Check sheet for the modelled part. Datum: model origin and axes. Units: mm. Face numbers are marked on the shaded views. A direction names the side the tool comes from. Coordinates: 2 decimals unless noted, no trailing zeros. Order: outer loops, then holes, each group sorted by start corner. A loop starts at its lowest first (then second) coordinate and runs counter-clockwise, first axis right, second up.
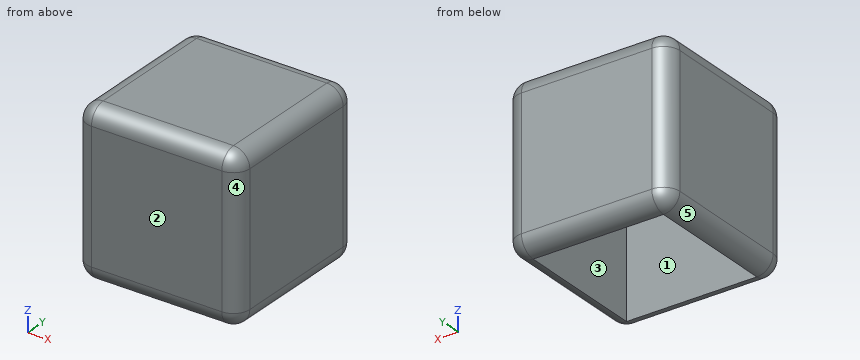
from build123d import *

# Parameters (mm, degrees)
F0_W      = 101.6
F0_H      = 101.6
F1_DEPTH  = 101.6
F2_R      = 50.8
F3_DEPTH  = 101.6
F9_W      = 101.6
F9_H      = 101.6
F10_DEPTH = 101.6
F11_R     = 10.16
F12_W     = 81.28
F12_H     = 81.28
F14_DEPTH = 88.9


# Not quite as in the source:
# - a feature of the source that left no trace in its solid (it failed there, or was rolled back) is left out


with BuildPart() as f1:
    # F0 (on Top) → F1 (new body)
    with BuildSketch(Plane.XY):
        Rectangle(F0_W, F0_H)
    extrude(amount=F1_DEPTH)


with BuildPart() as f3:
    # F2 (on Top) → F3 (new body)
    with BuildSketch(Plane.XY):
        Circle(F2_R)
    extrude(amount=F3_DEPTH)


with BuildPart() as f5:
    # F4 (on Front) → F5 (revolve)
    with BuildSketch(Plane.XZ):
        with BuildLine():
            Line((-42.8895973013, 27.2235641188), (42.8895973013, -27.2235641188))
            ThreePointArc((42.8895973013, -27.2235641188), (27.2235641188, 42.8895973013), (-42.8895973013, 27.2235641188))
        make_face()
    revolve(axis=Axis((0, 0, 0), (0.8442834114, 0, -0.5358969315)))


with BuildPart() as f10:
    # F9 (on Top) → F10 (new body)
    with BuildSketch(Plane.XY):
        Rectangle(F9_W, F9_H)
    extrude(amount=F10_DEPTH)

    # F11
    f11_edges = [f10.edges().sort_by_distance(p)[0] for p in [
        (-50.8, 50.8, 50.8),
        (-50.8, 0, 101.6),
        (0, 50.8, 101.6),
        (50.8, 0, 101.6),
        (50.8, 50.8, 50.8),
        (50.8, -50.8, 50.8),
        (50.8, 0, 0),
        (0, -50.8, 0),
        (-50.8, -50.8, 50.8),
        (-50.8, 0, 0),
        (0, 50.8, 0),
        (0, -50.8, 101.6),
    ]]
    fillet(f11_edges, radius=F11_R)

    # F12 (on face) → F14 (cut)
    with BuildSketch(Plane(origin=(0, 0, 0), x_dir=(1, 0, 0), z_dir=(0, 0, -1))):
        Rectangle(F12_W, F12_H)
    extrude(amount=-F14_DEPTH, mode=Mode.SUBTRACT)


solid = f10.part
(1) Go/stop test with a flat-tipped pin: P1, Ø6, axis at x = 25, y = -34, coming from the -Z side. Record where the tip stops, or that it passes through.
Filled in:
P1: stops at z = 88.9
(2) Release check for a two-part mould opening along Y. For the marked faces 3, 4 and 5 record: +Y half, -Y half, draft (parallel to the pull), parting line (faces both ways), or undercut.
Filled in:
face 3: undercut
face 4: -Y half
face 5: draft
(3) Cross-section at A-A (z = 27). Enter the section's corners in (x, y), and give its area (3 significant figures).
Filled in:
outline: (-50.8, -40.64) arc R10.16 ccw to (-40.64, -50.8) - (40.64, -50.8) arc R10.16 ccw to (50.8, -40.64) - (50.8, 40.64) arc R10.16 ccw to (40.64, 50.8) - (-40.64, 50.8) arc R10.16 ccw to (-50.8, 40.64) - close; hole (-40.64, -40.64) - (40.64, -40.64) - (40.64, 40.64) - (-40.64, 40.64) - close
area: 3,630 mm2
(4) Thickness scan on probe 1 along Y at (x, z) = (39, 38); probe 2 along Z at (x, y) = (36, 37.5). Record the ranges inside material, lowest first.
Filled in:
probe 1: y = -50.8 to -40.64, 40.64 to 50.8
probe 2: z = 88.9 to 101.6
(5) Cross-section at D-D (x = 43.5). Enter the section's corners in (y, z), and give its area (3 significant figures).
Filled in:
outline: (-50.39, 10.16) arc R9.75 ccw to (-40.64, 0.41) - (40.64, 0.41) arc R9.75 ccw to (50.39, 10.16) - (50.39, 91.44) arc R9.75 ccw to (40.64, 101.19) - (-40.64, 101.19) arc R9.75 ccw to (-50.39, 91.44) - close
area: 10,100 mm2
(6) Tool access check on the marked faces 1 and 2. Record the directions out of +Z, -Z, +X, -X, +Y, -Y that give a thin tool (end or side, any length) a straight path to the whole face; none if there is none.
Filled in:
face 1: -Z
face 2: +Z, -Z, +X, -X, -Y
(7) Cross-section at B-B (y = -30). Enter the section's corners in (x, z).
Filled in:
outline: (-50.8, 10.16) arc R10.16 ccw to (-40.64, 0) - (-40.64, 88.9) - (40.64, 88.9) - (40.64, 0) arc R10.16 ccw to (50.8, 10.16) - (50.8, 91.44) arc R10.16 ccw to (40.64, 101.6) - (-40.64, 101.6) arc R10.16 ccw to (-50.8, 91.44) - close
